Study the drawing (mm; zero at the part's minimum x, y, z) and answer. A direction names the side the tool comes from. Round coordinates to 2 decimals unless told otherwise and drop trailing zeros. Loops run counter-clockwise (first coordinate to the right, second up) from the corner with the lowest first, then second, coordinate; pieces in that order, holes last. Notation, with made-up numbers: (25.5, -22) -> (82.5, -22) arc R4 cw to (82.5, -15) -> close; hole circle Ø4 at (-1, 32). An arc over 180 degrees is marked (long way). Write each question's results on one line, items separated by ' | '. Start each with the question number.
(1) A flat-ended cylindrical pin translates along its axis: pin 1 (2.5 mm diameter, centred on x = 3.8, y = 5, fed in from +Z). Find the tip coordinate at first contact, or state that the pin passes through.
(2) The part is cut by section B-B (x = 11.8). Determine the outline of the cut face in (y, z).
(3) The part is cut by section D-D (y = 7). Determine the outline of the cut face in (x, z).
(4) The part is cut by section A-A (y = 5). Determine the outline of the cut face in (x, z).
(5) Determine the mould class of the marked faces 1, 2 and 3 for opening direction Y: released by +Y, released by -Y, zero draft, split by the parting line, or undercut.
(6) For the marked faces 4 and 5, determine the directions among +Z, -Z, +X, -X, +Y, -Y from which every point of the face is accessible in a straight line to the end or side of a thin tool.
(7) Straight lines are drawn through the part: probe 1 along Y at (x, z) = (11.8, 2.9); probe 2 along Y at (x, z) = (19.8, 2.85); probe 3 along Z at (x, y) = (15.25, 2). For each, find the intervals that lie inside material, in ascending order.
(8) The part is cut by section C-C (z = 1.3). Determine the outline of the cut face in (x, y), plus the area to 3 significant figures.
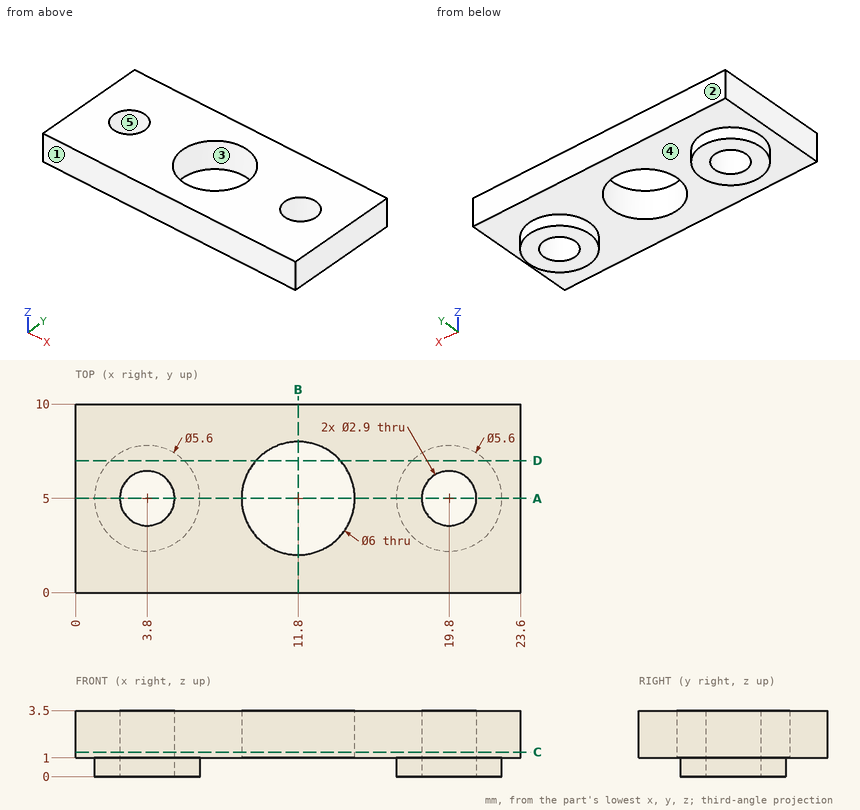
Checked values:
1) pin 1: passes through
2) outline: (0, 1) -> (2, 1) -> (2, 3.5) -> (0, 3.5) -> close; (8, 1) -> (10, 1) -> (10, 3.5) -> (8, 3.5) -> close
3) outline: (0, 1) -> (1.84, 1) -> (1.84, 0) -> (5.76, 0) -> (5.76, 1) -> (9.56, 1) -> (9.56, 3.5) -> (0, 3.5) -> close; (14.04, 1) -> (17.84, 1) -> (17.84, 0) -> (21.76, 0) -> (21.76, 1) -> (23.6, 1) -> (23.6, 3.5) -> (14.04, 3.5) -> close
4) outline: (0, 1) -> (1, 1) -> (1, 0) -> (2.35, 0) -> (2.35, 3.5) -> (0, 3.5) -> close; (5.25, 0) -> (6.6, 0) -> (6.6, 1) -> (8.8, 1) -> (8.8, 3.5) -> (5.25, 3.5) -> close; (14.8, 1) -> (17, 1) -> (17, 0) -> (18.35, 0) -> (18.35, 3.5) -> (14.8, 3.5) -> close; (21.25, 0) -> (22.6, 0) -> (22.6, 1) -> (23.6, 1) -> (23.6, 3.5) -> (21.25, 3.5) -> close
5) face 1: released by -Y | face 2: released by +Y | face 3: undercut
6) face 4: -Z | face 5: +Z, -Z
7) probe 1: y = 0 to 2, 8 to 10 | probe 2: y = 0 to 3.55, 6.45 to 10 | probe 3: z = 1 to 3.5
8) outline: (0, 0) -> (23.6, 0) -> (23.6, 10) -> (0, 10) -> close; hole circle Ø2.9 at (3.8, 5); hole circle Ø6 at (11.8, 5); hole circle Ø2.9 at (19.8, 5) | area: 195 mm2
